```python
from build123d import *

# Parameters (mm, degrees)
SKETCH_1_R               = 3
EXTRUDE_1_DEPTH          = 15
SKETCH_2_R               = 3
CUT_EXTRUDE_1_DEPTH      = 30
MIRROR_2_COPY_1_SKETCH_R = 3
MIRROR_2_COPY_1_DEPTH    = 30
CUT_EXTRUDE_2_DEPTH      = 4.5
MIRROR_4_COPY_1_DEPTH    = 4.5


with BuildPart() as part:
    # 草图1 → 凸台-拉伸1 (new body)
    with BuildSketch(Plane.XY):
        Polygon((-115, 229), (-115, -229), (-85, -229), (-85, -19), (85, -19), (85, -229), (115, -229), (115, 229), (85, 229), (85, 19), (-85, 19), (-85, 229), align=None)
        Circle(SKETCH_1_R, mode=Mode.SUBTRACT)
        with Locations((50, 0)):
            Circle(SKETCH_1_R, mode=Mode.SUBTRACT)
        with Locations((100, 0)):
            Circle(SKETCH_1_R, mode=Mode.SUBTRACT)
        with Locations((-50, 0)):
            Circle(SKETCH_1_R, mode=Mode.SUBTRACT)
        with Locations((-100, 0)):
            Circle(SKETCH_1_R, mode=Mode.SUBTRACT)
        with Locations((100, 50)):
            Circle(SKETCH_1_R, mode=Mode.SUBTRACT)
        with Locations((100, 100)):
            Circle(SKETCH_1_R, mode=Mode.SUBTRACT)
        with Locations((100, 150)):
            Circle(SKETCH_1_R, mode=Mode.SUBTRACT)
        with Locations((-100, -50)):
            Circle(SKETCH_1_R, mode=Mode.SUBTRACT)
        with Locations((-100, -100)):
            Circle(SKETCH_1_R, mode=Mode.SUBTRACT)
        with Locations((-100, -150)):
            Circle(SKETCH_1_R, mode=Mode.SUBTRACT)
        with Locations((100, -50)):
            Circle(SKETCH_1_R, mode=Mode.SUBTRACT)
        with Locations((100, -100)):
            Circle(SKETCH_1_R, mode=Mode.SUBTRACT)
        with Locations((100, -150)):
            Circle(SKETCH_1_R, mode=Mode.SUBTRACT)
        with Locations((-100, 50)):
            Circle(SKETCH_1_R, mode=Mode.SUBTRACT)
        with Locations((-100, 100)):
            Circle(SKETCH_1_R, mode=Mode.SUBTRACT)
        with Locations((-100, 150)):
            Circle(SKETCH_1_R, mode=Mode.SUBTRACT)
    extrude(amount=EXTRUDE_1_DEPTH)

    # 草图2 → 切除-拉伸1 (cut)
    with BuildSketch(Plane(origin=(0, 229, 0), x_dir=(1, 0, 0), z_dir=(0, 1, 0))):
        with Locations(Location((-100, -7.5, 0), (0, 0, 270))):
            Circle(SKETCH_2_R)
    cut_extrude_1 = extrude(amount=-CUT_EXTRUDE_1_DEPTH, mode=Mode.SUBTRACT)

    # 镜向1: 切除-拉伸1 across plane
    add(cut_extrude_1.mirror(Plane.ZX), mode=Mode.SUBTRACT)

    # 镜向2: 切除-拉伸1 across plane
    add(cut_extrude_1.mirror(Plane(origin=(0, 0, 0), x_dir=(0, 0, 1), z_dir=(1, 0, 0))), mode=Mode.SUBTRACT)

    # 镜向2 copy 1 sketch → 镜向2 copy 1 (cut)
    with BuildSketch(Plane(origin=(0, -229, 0), x_dir=(-1, 0, 0), z_dir=(0, -1, 0))):
        with Locations(Location((-100, -7.5, 0), (0, 0, 270))):
            Circle(MIRROR_2_COPY_1_SKETCH_R)
    extrude(amount=-MIRROR_2_COPY_1_DEPTH, mode=Mode.SUBTRACT)

    # 草图3 → 切除-拉伸2 (cut)
    with BuildSketch(Plane(origin=(0, 209, 0), x_dir=(1, 0, 0), z_dir=(0, 1, 0))):
        Polygon((-104.25, -9.585865128), (-104.25, -15), (-95.75, -15), (-95.75, -9.783166039), (-95.75, -5.046261356), (-100, -2.592522712), (-104.25, -5.046261356), align=None)
    cut_extrude_2 = extrude(amount=CUT_EXTRUDE_2_DEPTH, mode=Mode.SUBTRACT)

    # 镜向3: 切除-拉伸2 across plane
    add(cut_extrude_2.mirror(Plane.ZX), mode=Mode.SUBTRACT)

    # 镜向4: 切除-拉伸2 across plane
    add(cut_extrude_2.mirror(Plane(origin=(0, 0, 0), x_dir=(0, 0, 1), z_dir=(1, 0, 0))), mode=Mode.SUBTRACT)

    # 镜向4 copy 1 sketch → 镜向4 copy 1 (cut)
    with BuildSketch(Plane(origin=(0, -209, 0), x_dir=(-1, 0, 0), z_dir=(0, -1, 0))):
        Polygon((-104.25, -9.585865128), (-104.25, -15), (-95.75, -15), (-95.75, -9.783166039), (-95.75, -5.046261356), (-100, -2.592522712), (-104.25, -5.046261356), align=None)
    extrude(amount=MIRROR_4_COPY_1_DEPTH, mode=Mode.SUBTRACT)


solid = part.part
```
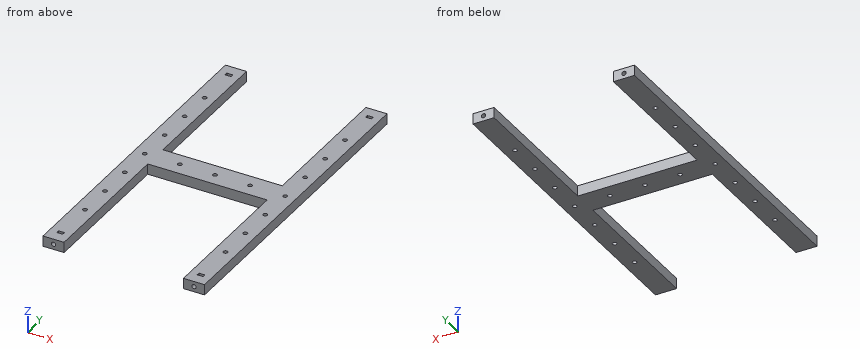
The model under review builds one solid part; all positions refer to its coordinate system, in mm. Round coordinates to 2 decimals unless told otherwise and drop trailing zeros. Order: outer loops, then holes, each group sorted by start corner. A loop starts at its lowest first (then second) coordinate and runs counter-clockwise, first axis right, second up.
(1) Take a section at A-A, the plane y = 122. State the section outline as (x, z) points.
Working result:
outline: (-115, 0) - (-85, 0) - (-85, 15) - (-115, 15) - close; (85, 0) - (115, 0) - (115, 15) - (85, 15) - close
(2) Wall thickness on L1, parallel to X at y = -150, z = 6.5; L2, parallel to Z at x = 100, y = -204; L3, parallel to X at y = -104.5, z = 3: over which ranges is each line inside the solid? List them lowest first.
Working result:
L1: x = -115 to -103, -97 to -85, 85 to 97, 103 to 115
L2: z = 0 to 4.5, 10.5 to 15
L3: x = -115 to -85, 85 to 115
(3) For P1, Ø2.5, axis at x = 101, z = 7.5, coming from the +Y side; P2, Ø3.5, axis at x = 100, z = 7.5, coming from the -Y side; P3, Ø6, axis at x = 78.5, z = 6.5, coming from the +Y side, all flat-tipped, find the tip position at first contact; note any pin that passes through.
Working result:
P1: stops at y = 199
P2: stops at y = -199
P3: stops at y = 19
(4) Take a section at B-B, the plane x = 77.5. State the section outline as (y, z) points, plus the area to 3 significant figures.
Working result:
outline: (-19, 0) - (19, 0) - (19, 15) - (-19, 15) - close
area: 570 mm2
